```python
from build123d import *

# Parameters (mm, degrees)
F0_W       = 63.5
F0_H       = 38.1
F1_DEPTH   = 279.4
F2_SIZE2   = 76.19999
F2_SIZE    = 38.09999
F2_2_SIZE2 = 76.19999
F2_2_SIZE  = 38.09999


# Not quite as in the source:
# - a fillet or chamfer is up to 0.001 mm smaller than in the source, because OpenCascade refuses the exact size


with BuildPart() as f1:
    # F0 (on Front) → F1 (new body)
    with BuildSketch(Plane.XZ):
        with Locations((-31.75, -19.05)):
            Rectangle(F0_W, F0_H)
        Polygon((0, 0), (0, -38.1), (139.7, -38.1), (63.5, 0), align=None)
        Polygon((-63.5, 0), (-139.7, -38.1), (-63.5, -38.1), align=None)
    extrude(amount=F1_DEPTH)

    # F2 (size 38.1 and 76.2 in the source; OpenCascade refuses exactly that, so slightly less here)
    f2_edges = [f1.edges().sort_by_distance(p)[0] for p in [
        (0, -279.4, 0),
    ]]
    f2_side = f1.faces().sort_by_distance((0, -279.4, -21.43125))[0]
    chamfer(f2_edges, length=F2_SIZE, length2=F2_SIZE2, reference=f2_side)

    # F2#2 (size 38.1 and 76.2 in the source; OpenCascade refuses exactly that, so slightly less here)
    f2_2_edges = [f1.edges().sort_by_distance(p)[0] for p in [
        (0, 0, 0),
    ]]
    f2_2_side = f1.faces().sort_by_distance((0, 0, -21.43125))[0]
    chamfer(f2_2_edges, length=F2_2_SIZE, length2=F2_2_SIZE2, reference=f2_2_side)


solid = f1.part
```
Check sheet for the modelled part. Datum: model origin and axes. Units: mm. Round coordinates to 2 decimals unless told otherwise and drop trailing zeros. Loops run counter-clockwise (first coordinate to the right, second up) from the corner with the lowest first, then second, coordinate; pieces in that order, holes last. Notation, with made-up numbers: M 87.25,2.5 L 140.25,2.5 A31 cw 140.25,31.5 Z; hole C 28.5,-19 d6. An arc over 180 degrees is marked long. Answer as a JSON object with one key per item and string values.
1. Section check C-C (z = -28). Record the boundary of the cut face in (x, y), plus the area to 3 significant figures.
Reply:
{"outline": "M -119.5,-259.2 L 119.5,-259.2 L 119.5,-20.2 L -119.5,-20.2 Z", "area": "57,100 mm²"}
2. Gauge pin test, flat ends, axial feed: P1, Ø4, axis at x = -13.5, z = -5.5, coming from the +Y side; P2, Ø5, axis at y = -132, z = -26, coming from the +X side; P3, Ø4, axis at x = -101.5, y = -241, coming from the +Z side. Record the tip position at first contact, or that the pin passes through.
Reply:
{"P1": "stops at y = -61.2", "P2": "stops at x = 120.5", "P3": "stops at z = -18.24"}
3. Scan lines: line 1 (Z direction, x = -82, y = -100); line 2 (Z direction, x = 71.5, y = -159); line 3 (X direction, y = -194.5, z = -27.5). Record each from-to range of solid material in increasing order.
Reply:
{"line 1": "z = -38.1 to -9.25", "line 2": "z = -38.1 to -4", "line 3": "x = -118.5 to 118.5"}
4. Section check A-A (y = -128.5). Record the boundary of the cut face in (x, z).
Reply:
{"outline": "M -139.7,-38.1 L 139.7,-38.1 L 63.5,0 L -63.5,0 Z"}
